Read the model definition and answer for the solid it produces. Units are mm, in the model's axes. Face numbers are marked on the shaded views. A direction names the side the tool comes from. Coordinates: 2 decimals unless noted, no trailing zeros. Order: outer loops, then holes, each group sorted by start corner. A loop starts at its lowest first (then second) coordinate and runs counter-clockwise, first axis right, second up. Notation, with made-up numbers: M 42,10.25 L 92,10.25 A23 ccw 92,33.25 Z; hole C -15.5,41.5 d3. An arc over 180 degrees is marked long. Put each result on its own line as item: value.
Autodesk Fusion 360 part; units mm, degrees
sketch "Skizze1" plane through (0, 0, 0) normal (0, 0, 1) x (1, 0, 0)
  circle A0 centre (0, 0) radius 17
  dimension "d1" = 34
extrude "Extrusion1" add sketch "Skizze1" along normal blind 5
sketch "Skizze2" plane through (0, 0, 5) normal (0, 0, 1) x (-1, 0, 0)
  circle A0 centre (0, 0) radius 17
  circle A1 centre (0, 0) radius 20
  dimension "d5" = 40
extrude "Extrusion2" add sketch "Skizze2" along normal blind 2 contours A0 | A1
sketch "Skizze3" plane through (0, 0, 0) normal (0, 0, -1) x (1, 0, 0)
  circle A0 centre (0, 0) radius 17
  circle A1 centre (0, 0) radius 20
  dimension "d8" = 40
extrude "Extrusion3" add sketch "Skizze3" along normal blind 2 contours A0 | A1
sketch "Skizze4" plane through (0, 0, 7) normal (0, 0, 1) x (-1, 0, 0)
  circle A0 centre (0, 0) radius 20
  circle A1 centre (0, 0) radius 13.05
  dimension "d11" = 26.1
extrude "Extrusion4" cut sketch "Skizze4" against normal blind 23 contours A1
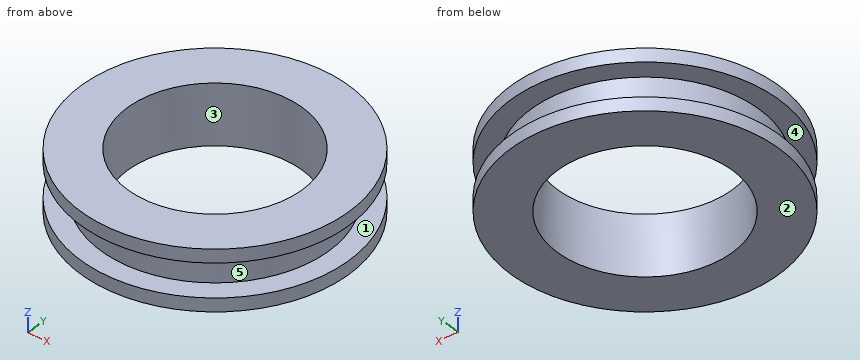
Q1. Find section A-A on x = 0. Write down the section's boundary in (y, z), plus the area to 3 significant figures.
Answers below:
outline: M -20,-2 L -13.05,-2 L -13.05,7 L -20,7 L -20,5 L -17,5 L -17,0 L -20,0 Z; M 13.05,-2 L 20,-2 L 20,0 L 17,0 L 17,5 L 20,5 L 20,7 L 13.05,7 Z
area: 95.1 mm^2
Q2. Given pin 1 (1.5 mm diameter, centred on x = 8, z = 5, fed in from +Y); pin 2 (15.5 mm diameter, centred on x = 0, y = 0, fed in from +Z); pin 3 (5 mm diameter, centred on x = 11.5, z = -1, fed in from +Y); pin 4 (2 mm diameter, centred on y = 9, z = 5.5, fed in from +X), each flat-ended and moving along its own axis, determine where each tip first touches the part or whether it passes through.
Answers below:
pin 1: stops at y = 18.64
pin 2: passes through
pin 3: stops at y = 17.86
pin 4: stops at x = 18.33
Q3. For a pull along X with two mould halves and no side action, classify the marked faces 3, 4 and 5 as +X half, -X half, draft (parallel to the pull), parting line (faces both ways), or undercut.
Answers below:
face 3: undercut
face 4: draft
face 5: parting line
Q4. A tool of negligible diameter and unlimited length cuts with its end or side. For the marked faces 1 and 2, from which of +Z, -Z, +X, -X, +Y, -Y can it reach the whole face along a straight path? Write none if from no direction.
Answers below:
face 1: none
face 2: -Z, +X, -X, +Y, -Y
Q5. Find section C-C on z = -1.5. Write down the section's boundary in (x, y).
Answers below:
outline: C 0,0 d40; hole C 0,0 d26.1
Q6. Find section D-D on x = -16.5. Write down the section's boundary in (y, z).
Answers below:
outline: M -11.3,-2 L 11.3,-2 L 11.3,0 L 4.09,0 L 4.09,5 L 11.3,5 L 11.3,7 L -11.3,7 L -11.3,5 L -4.09,5 L -4.09,0 L -11.3,0 Z
Q7. Consider line 1 along Y through (x, z) = (0, 4); line 2 along X through (y, z) = (0, 5.25); line 3 along Z through (x, y) = (-9, 17). Determine where each line is inside the solid, lowest interval first.
Answers below:
line 1: y = -17 to -13.05, 13.05 to 17
line 2: x = -20 to -13.05, 13.05 to 20
line 3: z = -2 to 0, 5 to 7
